Input: part model. Units: mm. Frame: model coordinates. A direction names the side the tool comes from. Give positions to 0.01 mm unless a question says otherwise; leave off trailing zeros. Order: outer loops, then holes, each group sorted by start corner. A loop starts at its lowest first (then second) coordinate and runs counter-clockwise, first axis right, second up. Notation, with made-up numbers: (60.25, 20.25) - (93.25, 20.25) arc R25 ccw to (93.25, 45.25) - close; hole circle Ø5 at (24.5, -29). An arc over 180 degrees is marked (long way). Answer in a Markdown table with one row per item. Add a question column.
from build123d import *

# Parameters (mm, degrees)
CROQUIS1_W              = 51
CROQUIS1_H              = 52
SALIENTE_EXTRUIR1_DEPTH = 1
CROQUIS2_W              = 30
CROQUIS2_H              = 26
CROQUIS2_W_2            = 3.538114814
CROQUIS2_H_2            = 7.817941565
CROQUIS2_W_3            = 2.595962414
SALIENTE_EXTRUIR2_DEPTH = 3
CROQUIS3_W              = 51
CROQUIS3_H              = 1
CORTAR_EXTRUIR2_DEPTH   = 3


with BuildPart() as part:
    # Croquis1 → Saliente-Extruir1 (new body)
    with BuildSketch(Plane.XY):
        with Locations((25.5, -26)):
            Rectangle(CROQUIS1_W, CROQUIS1_H)
    extrude(amount=SALIENTE_EXTRUIR1_DEPTH)

    # Croquis2 → Saliente-Extruir2 (add)
    with BuildSketch(Plane.XY.offset(1)):
        with Locations((36, -31)):
            Rectangle(CROQUIS2_W, CROQUIS2_H)
        with Locations((57.769057407, -33.036147408)):
            Rectangle(CROQUIS2_W_2, CROQUIS2_H_2)
        with Locations((54.702018793, -33.036147408)):
            Rectangle(CROQUIS2_W_3, CROQUIS2_H_2)
        Polygon((56, -18), (51, -18), (51, -44), (56, -44), (56, -36.945118191), (53.404037586, -36.945118191), (53.404037586, -29.127176626), (56, -29.127176626), align=None)
    extrude(amount=SALIENTE_EXTRUIR2_DEPTH)

    # Croquis3 → Cortar-Extruir2 (cut)
    with BuildSketch(Plane.XY.offset(1)):
        with Locations((25.5, -0.5)):
            Rectangle(CROQUIS3_W, CROQUIS3_H)
    extrude(amount=-CORTAR_EXTRUIR2_DEPTH, mode=Mode.SUBTRACT)


solid = part.part
Q1. Section A-A, the plane z = 3.1. Return loops of the section in (x, y), then the cut area to 3 significant figures.
Q2. Access query for faces 1 (the flat face through (56, -24, 2)), 2 (the flat face through (54, -31, 1)), 3 (the flat face through (58, -36.945, 2)), 4 (the flat face through (21, -31, 2)). Directions: +Z, -Z, +X, -X, +Y, -Y. A direction counts if a zero-diameter tool reaches every point of the face in a straight line with its end or side. Return the directions, or none.
Q3. Line query: probe 1 along Y at (x, z) = (29, 2.55); probe 2 along X at (y, z) = (-47.5, 0.9); probe 3 along Z at (x, y) = (14.5, -3.5). Output: solid intervals per line, ascending.
Q4. Section C-C, the plane x = 52. Return loops of the section in (y, z).
Q5. Contact query for flat-ended pins moving along their axis: P1, Ø0.9, axis at x = 57.5, z = 3, coming from the +Y side; P2, Ø0.9, axis at y = -22.5, z = 2, coming from the +X side; P3, Ø0.5, axis at y = -25.5, z = 0.5, coming from the +X side. Output: stop coordinate, or through.
Q6. Section B-B, the plane y = -33. Return loops of the section in (x, z), then the cut area to 3 significant figures.
Q7. Section D-D, the plane x = 15.5. Return loops of the section in (y, z), then the cut area to 3 significant figures.
Computed:
| question | item | result |
|---|---|---|
| 1 | outline | (21, -44) - (56, -44) - (56, -36.95) - (59.54, -36.95) - (59.54, -29.13) - (56, -29.13) - (56, -18) - (21, -18) - close |
| 1 | area | 938 mm^2 |
| 2 | face 1 | +Z, -Z, +X, +Y |
| 2 | face 2 | -Z, +X, +Y, -Y |
| 2 | face 3 | +Z, -Z, +X, -Y |
| 2 | face 4 | +Z, -X, +Y, -Y |
| 3 | probe 1 | y = -44 to -18 |
| 3 | probe 2 | x = 0 to 51 |
| 3 | probe 3 | z = 0 to 1 |
| 4 | outline | (-44, 1) - (-18, 1) - (-18, 4) - (-44, 4) - close |
| 5 | P1 | stops at y = -29.13 |
| 5 | P2 | stops at x = 56 |
| 5 | P3 | stops at x = 51 |
| 6 | outline | (0, 0) - (51, 0) - (51, 1) - (59.54, 1) - (59.54, 4) - (21, 4) - (21, 1) - (0, 1) - close |
| 6 | area | 167 mm^2 |
| 7 | outline | (-52, 0) - (-1, 0) - (-1, 1) - (-52, 1) - close |
| 7 | area | 51.0 mm^2 |
